Design review of the part shown in the three views and the two pictorial views. Dimensions are in mm from the part's minimum x, y and z. A direction names the side the tool comes from. Round coordinates to 2 decimals unless told otherwise and drop trailing zeros. Loops run counter-clockwise (first coordinate to the right, second up) from the corner with the lowest first, then second, coordinate; pieces in that order, holes last. Notation, with made-up numbers: (-29.5, 45.5) -> (26.5, 45.5) arc R13 cw to (26.5, 56.5) -> close; hole circle Ø2 at (2.25, 14.25). An arc over 180 degrees is marked (long way). Use a Markdown table: item, result. Add a question column.
1) Mouldability with a two-part tool opening along Y and no side actions: class the marked faces 1, 2, 3 and 4 as released by +Y, released by -Y, zero draft, split by the parting line, or undercut.
2) Consider section D-D on x = 19. State how many separate pieces and enclosed holes the cut face has, plus the area to 3 significant figures.
3) Wall thickness on probe 1 along Y at (x, z) = (14, 6.5); probe 2 along Y at (x, z) = (4, 12.5) (1 decimal); probe 3 along Z at (x, y) = (21, 92.5): over which ranges is each line inside the solid? List them lowest first.
4) Consider section B-B on y = 54. Give the boundary of the cut face in (x, z) (1 decimal).
5) Insertion check: pin 1 (4 mm diameter, centred on x = 17.5, z = 48, fed in from -Y); pin 2 (8 mm diameter, centred on x = 8, z = 53, fed in from -Y); pin 3 (14 mm diameter, centred on x = 13.5, y = 111, fed in from +Z). Each pin has a flat end and moves straight along its axis. Give the tip position at first contact, or say it passes through.
6) For the marked faces 5, 6 and 7, list the 3-axis set-ups (+Z, -Z, +X, -X, +Y, -Y) from which the entire face can be reached by the end or side of a thin tool; tool diameter is ignored.
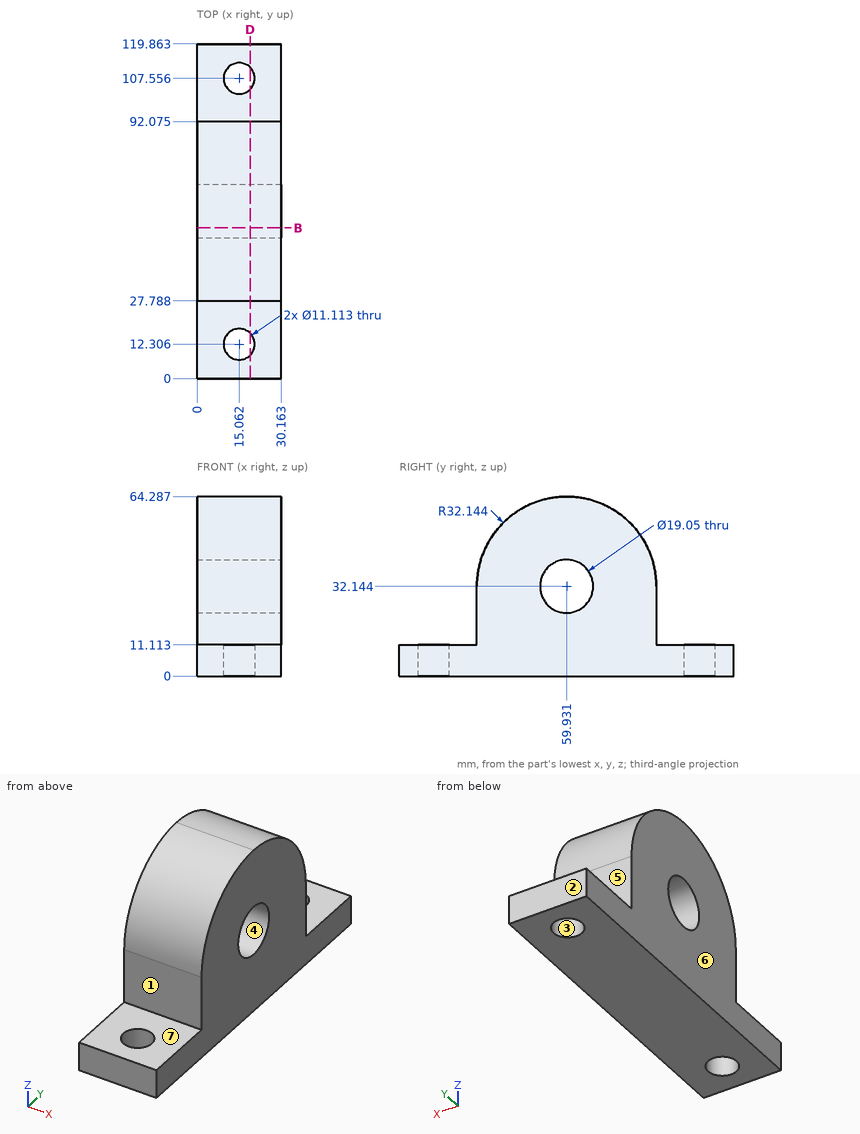
Result set:
| question | item | result |
|---|---|---|
| 1 | face 1 | released by -Y |
| 1 | face 2 | released by +Y |
| 1 | face 3 | undercut |
| 1 | face 4 | undercut |
| 2 | separate pieces | 3 |
| 2 | enclosed holes | 1 |
| 2 | area | 3,850 mm2 |
| 3 | probe 1 | 0 to 6.85, 17.76 to 102.1, 113.01 to 119.86 |
| 3 | probe 2 | 27.8 to 92.1 |
| 3 | probe 3 | 0 to 11.11 |
| 4 | outline | (0, 0) -> (30.2, 0) -> (30.2, 24.7) -> (0, 24.7) -> close; (0, 39.6) -> (30.2, 39.6) -> (30.2, 63.7) -> (0, 63.7) -> close |
| 5 | pin 1 | y = 30.93 |
| 5 | pin 2 | y = 32.56 |
| 5 | pin 3 | z = 11.11 |
| 6 | face 5 | +Z, +X, -X, +Y |
| 6 | face 6 | +Z, -Z, -X, +Y, -Y |
| 6 | face 7 | +Z, +X, -X, -Y |
